from build123d import *

# Parameters (mm, degrees)
SKETCH1_W           = 113
SKETCH1_H           = 88
BOSS_EXTRUDE1_DEPTH = 2.5
SKETCH1_3_W         = 113
SKETCH1_3_H         = 88
SKETCH1_3_W_2       = 108
SKETCH1_3_H_2       = 83
BOSS_EXTRUDE2_DEPTH = 12.5
CUT_EXTRUDE4_REACH  = 90
SKETCH2_W           = 13.04
SKETCH2_H           = 5.92
SKETCH2_W_2         = 10
SKETCH2_H_2         = 6.35
SKETCH4_R           = 2.5875
BOSS_EXTRUDE5_DEPTH = 2.5
SKETCH4_4_R         = 1.0875
BOSS_EXTRUDE6_DEPTH = 5
CUT_EXTRUDE5_START  = -10
CUT_EXTRUDE5_DEPTH  = 10


with BuildPart() as part:
    # Sketch1 → Boss-Extrude1 (new body)
    with BuildSketch(Plane(origin=(0, 0, 0), x_dir=(1, 0, 0), z_dir=(0, 1, 0))):
        with Locations((54, 41.5)):
            Rectangle(SKETCH1_W, SKETCH1_H)
    extrude(amount=BOSS_EXTRUDE1_DEPTH)

    # Sketch1<3> → Boss-Extrude2 (add)
    with BuildSketch(Plane(origin=(0, 0, 0), x_dir=(1, 0, 0), z_dir=(0, 1, 0))):
        with Locations((54, 41.5)):
            Rectangle(SKETCH1_3_W, SKETCH1_3_H)
        with Locations((54, 41.5)):
            Rectangle(SKETCH1_3_W_2, SKETCH1_3_H_2, mode=Mode.SUBTRACT)
    extrude(amount=BOSS_EXTRUDE2_DEPTH)

    # Sketch2 → Cut-Extrude4 (cut, up to next)
    with BuildSketch(Plane(origin=(0, 0, -85.5), x_dir=(-1, 0, 0), z_dir=(0, 0, -1)), mode=Mode.PRIVATE) as cut_extrude4_sk1:
        with Locations((-38.02, 9.54)):
            Rectangle(SKETCH2_W, SKETCH2_H)
    cut_extrude4_tool1 = extrude(cut_extrude4_sk1.sketch, amount=-CUT_EXTRUDE4_REACH, mode=Mode.PRIVATE) & part.part
    add(cut_extrude4_tool1.solids().sort_by_distance((38.02, 9.54, -85.5))[0], mode=Mode.SUBTRACT)
    # Sketch2 → Cut-Extrude4 (cut, up to next)
    with BuildSketch(Plane(origin=(0, 0, -85.5), x_dir=(-1, 0, 0), z_dir=(0, 0, -1)), mode=Mode.PRIVATE) as cut_extrude4_sk2:
        with Locations((-7.675, 9.325)):
            Rectangle(SKETCH2_W_2, SKETCH2_H_2)
    cut_extrude4_tool2 = extrude(cut_extrude4_sk2.sketch, amount=-CUT_EXTRUDE4_REACH, mode=Mode.PRIVATE) & part.part
    add(cut_extrude4_tool2.solids().sort_by_distance((7.675, 9.325, -85.5))[0], mode=Mode.SUBTRACT)

    # Sketch4 → Boss-Extrude5 (add)
    with BuildSketch(Plane(origin=(0, 2.5, 0), x_dir=(1, 0, 0), z_dir=(0, 1, 0))):
        with Locations((2.54, 69.625)):
            Circle(SKETCH4_R)
        with Locations((50.8, 68.355)):
            Circle(SKETCH4_R)
        with Locations((7.62, 17.555)):
            Circle(SKETCH4_R)
        with Locations((35.56, 17.555)):
            Circle(SKETCH4_R)
    extrude(amount=BOSS_EXTRUDE5_DEPTH)

    # Sketch4<4> → Boss-Extrude6 (add)
    with BuildSketch(Plane(origin=(0, 2.5, 0), x_dir=(1, 0, 0), z_dir=(0, 1, 0))):
        with Locations((2.54, 69.625)):
            Circle(SKETCH4_4_R)
        with Locations((50.8, 68.355)):
            Circle(SKETCH4_4_R)
        with Locations((7.62, 17.555)):
            Circle(SKETCH4_4_R)
        with Locations((35.56, 17.555)):
            Circle(SKETCH4_4_R)
    extrude(amount=BOSS_EXTRUDE6_DEPTH)

    # Sketch5 → Cut-Extrude5 (cut)
    with BuildSketch(Plane(origin=(0, 12.5, 0), x_dir=(1, 0, 0), z_dir=(0, 1, 0)).offset(CUT_EXTRUDE5_START)):
        with BuildLine():
            Line((101.25, 83), (104.75, 83))
            ThreePointArc((104.75, 83), (103, 84.75), (101.25, 83))
        make_face()
        with BuildLine():
            Line((56.75, 83), (60.25, 83))
            ThreePointArc((60.25, 83), (58.5, 84.75), (56.75, 83))
        make_face()
        with BuildLine():
            Line((108, 70.75), (108, 67.25))
            ThreePointArc((108, 67.25), (109.75, 69), (108, 70.75))
        make_face()
        with BuildLine():
            Line((108, 15.75), (108, 12.25))
            ThreePointArc((108, 12.25), (109.75, 14), (108, 15.75))
        make_face()
    extrude(amount=CUT_EXTRUDE5_DEPTH, mode=Mode.SUBTRACT)


solid = part.part
Input: part model. Units: mm. Frame: model coordinates. A direction names the side the tool comes from. Give positions to 0.01 mm unless a question says otherwise; leave off trailing zeros. Write each loop counter-clockwise with the first axis right and the second up, starting at its lowest first coordinate (ties: lowest second). Pieces come first, ordered by that corner, then holes.
Q1. Section A-A, the plane y = 11.25. Output: boundary loops of the cut face in (x, z) (3 decimals), plus the area to 3 significant figures.
Q2. First-contact query: P1, Ø1.1, axis at x = 7, z = -17.5, coming from the +Y side; P2, Ø3, axis at x = 5.5, z = -85, coming from the +Y side. Flat tips, straight axial feed; report the tip coordinate or a pass-through.
Q3. Material intervals for probe 1 along X at (y, z) = (9, -27); probe 2 along Z at (x, y) = (97.5, 7.5); probe 3 along Y at (x, z) = (14.5, -36.5), sorted ascending.
Q4. Set-up query: faces 4 (the face through (44.54, 9, -84)), 5 (the face through (109.75, 7.43, -68.96)), 6 (the face through (53, 0, -42)). Return all of +Z, -Z, +X, -X, +Y, -Y with unobstructed straight access to the full face (end or side cutting, diameter ignored); none if empty.
Q5. Pull-direction query (Z, two-part tool) for faces 1 (the face through (49.94, 6.23, -67.69)), 2 (the face through (53, 6, 2.5)), 3 (the face through (8, 6.15, -84)); classes: pulls with the +Z half, pulls with the -Z half, needs draft (parallel to the pull), parting line crosses it, or undercut.
Q6. Section D-D, the plane z = -50. Output: boundary loops of the cut face in (x, y).
Q7. Section C-C, the plane y = 3.75. State how many separate pieces and enclosed holes the cut face has, plus the area to 3 significant figures.
Q8. Section B-B, the plane x = 58.5. Output: boundary loops of the cut face in (y, z).
Filled in:
1. outline: (-2.5, -85.5) - (2.675, -85.5) - (2.675, -83) - (0, -83) - (0, 0) - (108, 0) - (108, -12.25) arc R1.75 cw to (108, -15.75) - (108, -67.25) arc R1.75 cw to (108, -70.75) - (108, -83) - (104.75, -83) arc R1.75 cw to (101.25, -83) - (60.25, -83) arc R1.75 cw to (56.75, -83) - (44.54, -83) - (44.54, -85.5) - (110.5, -85.5) - (110.5, 2.5) - (-2.5, 2.5) - close; (12.675, -85.5) - (31.5, -85.5) - (31.5, -83) - (12.675, -83) - close
1. area: 903 mm2
2. P1: stops at y = 7.5
2. P2: stops at y = 6.15
3. probe 1: x = -2.5 to 0, 108 to 110.5
3. probe 2: z = -85.5 to -83, 0 to 2.5
3. probe 3: y = 0 to 2.5
4. face 4: -Z, +Y
4. face 5: +Y
4. face 6: +Z, -Z, +X, -X, -Y
5. face 1: undercut
5. face 2: pulls with the +Z half
5. face 3: needs draft
6. outline: (-2.5, 0) - (110.5, 0) - (110.5, 12.5) - (108, 12.5) - (108, 2.5) - (0, 2.5) - (0, 12.5) - (-2.5, 12.5) - close
7. separate pieces: 4
7. enclosed holes: 1
7. area: 1,040 mm2
8. outline: (0, -85.5) - (12.5, -85.5) - (12.5, -84.75) - (2.5, -84.75) - (2.5, 0) - (12.5, 0) - (12.5, 2.5) - (0, 2.5) - close
